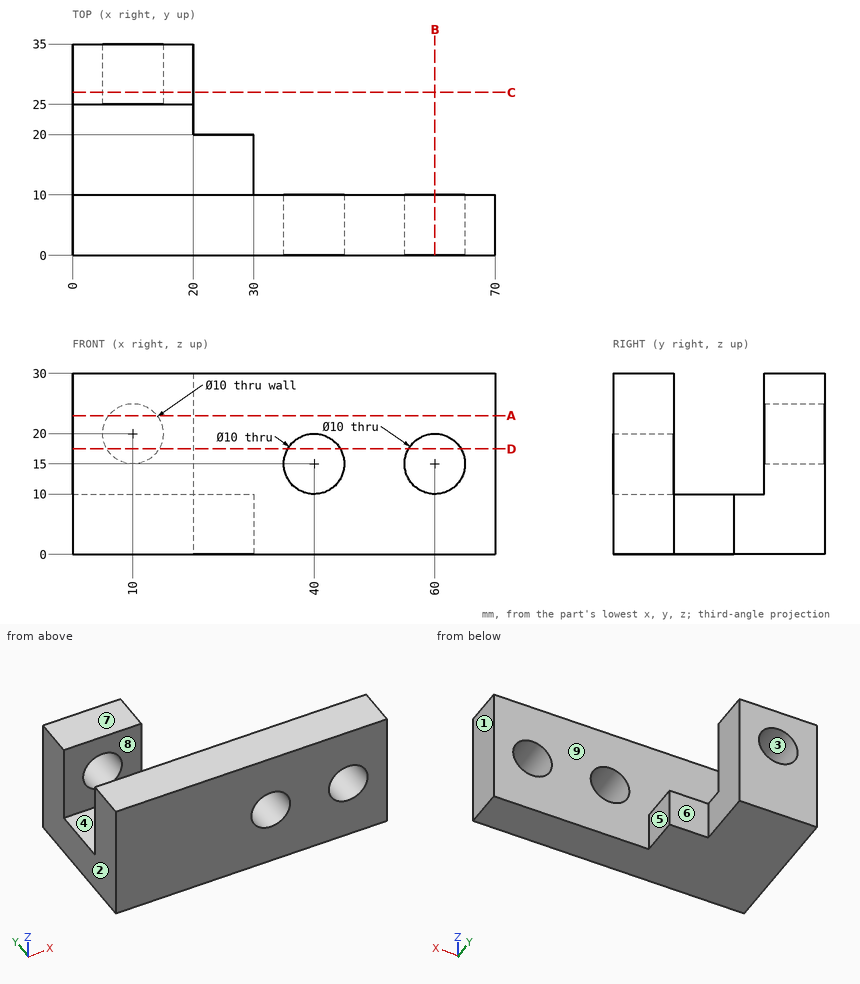
Can you work these out from the drawing? Everything is in mm from the part's minimum corner. A direction names the side the tool comes from. Round coordinates to 2 decimals unless told otherwise and drop trailing zeros. Order: outer loops, then holes, each group sorted by start corner. A loop starts at its lowest first (then second) coordinate and runs counter-clockwise, first axis right, second up. Notation, with made-up numbers: M 83.5,64 L 125.5,64 A26 cw 125.5,82 Z; hole C 77.5,9 d3. An arc over 180 degrees is marked long. Answer as CSV lines item,"result".
Item 1: Please list where these lines run through material, in increasing order: L1, parallel to X at y = 7.25, z = 15; L2, parallel to X at y = 28, z = 20; L3, parallel to Z at x = 40, y = 8.25. Write a range as [from, to].
From the geometry:
L1,"[0, 35], [45, 55], [65, 70]"
L2,"[0, 5], [15, 20]"
L3,"[0, 10], [20, 30]"
Item 2: Imagine slicing it at C-C on y = 27. List the corners of the cut face in (x, z) for me, and give its area (3 significant figures).
From the geometry:
outline,"M 0,0 L 20,0 L 20,30 L 0,30 Z; hole C 10,20 d10"
area,"521 mm2"
Item 3: Which directions (+Z, -Z, +X, -X, +Y, -Y) give clear straight access to the entire face, cutting with the end or side of a thin tool? Please do the marked faces 1, 2, 3, 4 and 5.
From the geometry:
face 1,"+Z, -Z, +X, +Y, -Y"
face 2,"+Z, -Z, -X, +Y, -Y"
face 3,"+Y"
face 4,"+Z, +X, -X"
face 5,"+Z, -Z, +X, +Y"
Item 4: We'd pull the mould along Y, two halves only. Please class the marked faces 6, 7, 8 and 9: +Y half, -Y half, draft (parallel to the pull), parting line (faces both ways), or undercut.
From the geometry:
face 6,"+Y half"
face 7,"draft"
face 8,"undercut"
face 9,"undercut"
Item 5: For pin 1 (11.5 mm diameter, centred on x = 60, z = 15, fed in from +Y); pin 2 (12 mm diameter, centred on y = 29.5, z = 8, fed in from +X); pin 3 (12 mm diameter, centred on y = 20.5, z = 5.5, fed in from +X), each with a flat end and sliding along its axis, tell me the tip position at first contact or that it passes through.
From the geometry:
pin 1,"y = 10"
pin 2,"x = 20"
pin 3,"x = 30"
Item 6: Imagine slicing it at B-B on x = 60. List the corners of the cut face in (y, z) for me, and give its area (3 significant figures).
From the geometry:
outline,"M 0,0 L 10,0 L 10,10 L 0,10 Z; M 0,20 L 10,20 L 10,30 L 0,30 Z"
area,"200 mm2"
Item 7: Imagine slicing it at A-A on z = 23. List the corners of the cut face in (x, y) for me, and give its area (3 significant figures).
From the geometry:
outline,"M 0,0 L 70,0 L 70,10 L 0,10 Z; M 0,25 L 6,25 L 6,35 L 0,35 Z; M 14,25 L 20,25 L 20,35 L 14,35 Z"
area,"820 mm2"
Item 8: Imagine slicing it at D-D on z = 17.5. List the corners of the cut face in (x, y) for me.
From the geometry:
outline,"M 0,0 L 35.67,0 L 35.67,10 L 0,10 Z; M 0,25 L 5.67,25 L 5.67,35 L 0,35 Z; M 14.33,25 L 20,25 L 20,35 L 14.33,35 Z; M 44.33,0 L 55.67,0 L 55.67,10 L 44.33,10 Z; M 64.33,0 L 70,0 L 70,10 L 64.33,10 Z"
